from build123d import *

# Parameters (mm, degrees)
F0_R = 10.915594


with BuildPart() as f2:
    # F2: sweep along a path in F1
    with BuildLine(Plane.XZ) as f2_path:
        Line((0, 0), (-110.754612, 0))
        ThreePointArc((-110.754612, 0), (-128.715125, 7.439488), (-136.154612, 25.4))
        Line((-136.154612, 25.4), (-136.154612, 139.267394))
        ThreePointArc((-136.154612, 139.267394), (-143.5941, 157.227906), (-161.554612, 164.667394))
        Line((-161.554612, 164.667394), (-241.116758, 164.667394))
    # F0 (on Right) → F2 (sweep)
    with BuildSketch(Plane.YZ):
        Circle(F0_R)
    sweep(path=f2_path.line)


solid = f2.part
Read the model definition and answer for the solid it produces. Units are mm, in the model's axes. A direction names the side the tool comes from. Give positions to 0.01 mm unless a question says otherwise; leave off trailing zeros. Loops run counter-clockwise (first coordinate to the right, second up) from the corner with the lowest first, then second, coordinate; pieces in that order, holes last. Notation, with made-up numbers: M 60,22 L 73,22 A11 cw 73,42 Z; hole C 58.5,54.25 d11. An arc over 180 degrees is marked long. Write each question's results on one line, items separated by ' | '.
1. Section A-A on x = -24 is taken. Give the vertices of the cut face in (y, z), plus the area to 3 significant figures.
Values:
outline: C 0,0 d21.83 | area: 374 mm^2
2. Straight lines are drawn through the part: line 1 (Z direction, x = -55, y = 1); line 2 (Z direction, x = -132.5, y = -3); line 3 (X direction, y = 9, z = 159.5). For each, find the intervals that lie inside material, in ascending order. Write a range as [from, to].
Values:
line 1: z = [-10.87, 10.87] | line 2: z = [-3.16, 160.35] | line 3: x = [-241.12, -137.31]
3. A tool of negligible diameter and unlimited length cuts with its end or side. For faces 1 (the face through (0, 0, 0)), 2 (the face through (-56.153, -2.366, 10.656)), from which of +Z, -Z, +X, -X, +Y, -Y can it reach the whole face along a straight path? Write none if from no direction.
Values:
face 1: +Z, -Z, +X, +Y, -Y | face 2: +X
4. Given pin 1 (8 mm diameter, centred on y = -3, z = 143.5, fed in from +X); pin 2 (3 mm diameter, centred on y = -3.5, z = 52.5, fed in from -X); pin 3 (5 mm diameter, centred on y = -2, z = 57, fed in from +X), each flat-ended and moving along its own axis, determine where each tip first touches the part or whether it passes through.
Values:
pin 1: stops at x = -125.27 | pin 2: stops at x = -146.89 | pin 3: stops at x = -125.24
